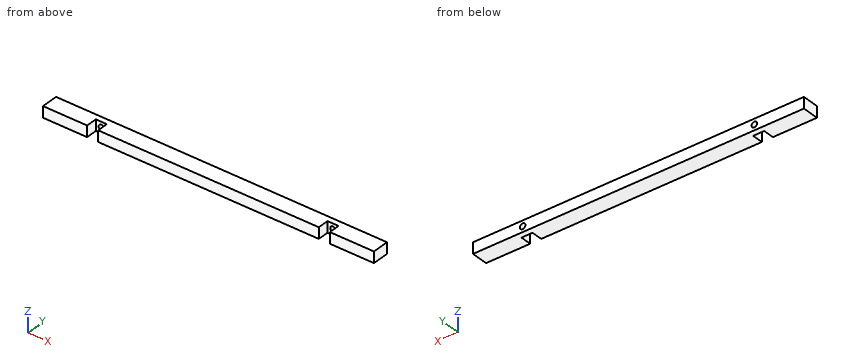
Autodesk Inventor part; units mm, degrees
ref_plane "YZ Plane" through (0, 0, 0) normal (1, 0, 0) x (0, 1, 0)
ref_plane "XZ Plane" through (0, 0, 0) normal (0, 1, 0) x (-1, 0, 0)
ref_plane "XY Plane" through (0, 0, 0) normal (0, 0, 1) x (1, 0, 0)
sketch "Sketch1" plane through (0, 0, 0) normal (0, 1, 0) x (-1, 0, 0)
  line L0 (0, 0) -> (381, 0)
  line L1 (381, 0) -> (381, -12.7)
  line L2 (381, -12.7) -> (0, -12.7)
  line L3 (0, -12.7) -> (0, 0)
  dimension "d0" = 381
  dimension "d1" = 12.7
extrude "Extrusion1" add sketch "Sketch1" along normal blind 19.05
sketch "Sketch2" plane through (0, 0, 0) normal (0, -1, 0) x (1, 0, 0)
  line L0 (-63.5, 0) -> (-50.8, 0)
  line L1 (-50.8, 0) -> (-50.8, -12.7)
  line L2 (-50.8, -12.7) -> (-63.5, -12.7)
  line L3 (-63.5, -12.7) -> (-63.5, 0)
  line L4 (0, -12.7) -> (0, 0)
  line L5 (-330.2, 0) -> (-317.5, 0)
  line L6 (-317.5, 0) -> (-317.5, -12.7)
  line L7 (-317.5, -12.7) -> (-330.2, -12.7)
  line L8 (-330.2, -12.7) -> (-330.2, 0)
  dimension "d4" = 12.7
  dimension "d5" = 12.7
  dimension "d6" = 50.8
  dimension "d7" = 12.7
  dimension "d8" = 12.7
  dimension "d9" = 330.2
extrude "Extrusion2" cut sketch "Sketch2" against normal blind 12.7
sketch "Sketch3" plane through (0, 19.05, 0) normal (0, 1, 0) x (1, 0, 0)
  circle A0 centre (-57.15, 6.35) radius 3.175
  line L0 (0, 0) -> (0, 12.7)
  line L1 (0, 12.7) -> (-381, 12.7)
  circle A1 centre (-323.85, 6.35) radius 3.175
  dimension "d12" = 6.35
  dimension "d13" = 57.15
  dimension "d15" = 6.35
  dimension "d16" = 6.35
  dimension "d17" = 323.85
hole "Hole1" at (-323.85, 19.05, -6.35) at (-57.15, 19.05, -6.35) direction (0, -1, 0) diameter 6.35 end through all
properties part number "Rack Side"
The listing builds one solid part. Answer for the finished solid, in the listing's coordinates (mm). Coordinates: 2 decimals unless noted, no trailing zeros. Loops run counter-clockwise (first coordinate to the right, second up) from the corner with the lowest first, then second, coordinate; pieces in that order, holes last. Notation, with made-up numbers: M 29,78.25 L 69,78.25 A15 ccw 69,97.25 Z; hole C 37.5,-7.5 d9. An arc over 180 degrees is marked long. Answer in a Markdown table with one row per item.
1) Find section A-A (z = -6.35). Determine the outline of the cut face in (x, y) (3 decimals).
Answers below:
| item | result |
|---|---|
| outline | M -381,0 L -330.2,0 L -330.2,12.7 L -327.025,12.7 L -327.025,19.05 L -381,19.05 Z; M -320.675,12.7 L -317.5,12.7 L -317.5,0 L -63.5,0 L -63.5,12.7 L -60.325,12.7 L -60.325,19.05 L -320.675,19.05 Z; M -53.975,12.7 L -50.8,12.7 L -50.8,0 L 0,0 L 0,19.05 L -53.975,19.05 Z |
2) Find the intervals of material crossed by probe 1 along X at (y, z) = (14, -6.35) (3 decimals); probe 2 along X at (y, z) = (7.5, -6.75); probe 3 along Z at (x, y) = (-57.15, 16.5) (3 decimals), in increasing order.
Answers below:
| item | result |
|---|---|
| probe 1 | -381 to -327.025, -320.675 to -60.325, -53.975 to 0 |
| probe 2 | -381 to -330.2, -317.5 to -63.5, -50.8 to 0 |
| probe 3 | -12.7 to -9.525, -3.175 to 0 |
3) Find section B-B (x = -57.15). Determine the outline of the cut face in (y, z) (3 decimals), then the cut area to 3 significant figures.
Answers below:
| item | result |
|---|---|
| outline | M 12.7,-12.7 L 19.05,-12.7 L 19.05,-9.525 L 12.7,-9.525 Z; M 12.7,-3.175 L 19.05,-3.175 L 19.05,0 L 12.7,0 Z |
| area | 40.3 mm^2 |
4) Find section C-C (y = 6.75). Determine the outline of the cut face in (x, z), then the cut area to 3 significant figures.
Answers below:
| item | result |
|---|---|
| outline | M -381,-12.7 L -330.2,-12.7 L -330.2,0 L -381,0 Z; M -317.5,-12.7 L -63.5,-12.7 L -63.5,0 L -317.5,0 Z; M -50.8,-12.7 L 0,-12.7 L 0,0 L -50.8,0 Z |
| area | 4,520 mm^2 |
5) Given pin 1 (6.5 mm diameter, centred on x = -324, z = -8, fed in from -Y), flat-ended and moving along its own axis, determine where the tip first touches the part or whether it passes through.
Answers below:
| item | result |
|---|---|
| pin 1 | y = 12.7 |
